Answer from the drawing. Dimensions are ordinates in mm from the lowest x, y and z of the part. A direction names the side the tool comes from. Give positions to 0.01 mm unless a question says otherwise; leave off trailing zeros. Write each loop counter-clockwise with the first axis right and the second up, starting at its lowest first coordinate (ties: lowest second). Pieces come first, ordered by that corner, then holes. Notation, with made-up numbers: M 23.5,50 L 48.5,50 A13 ccw 48.5,68 Z; hole C 9.5,37.5 d7. An arc over 180 degrees is marked long. Answer as a JSON object with one key per item and string values.
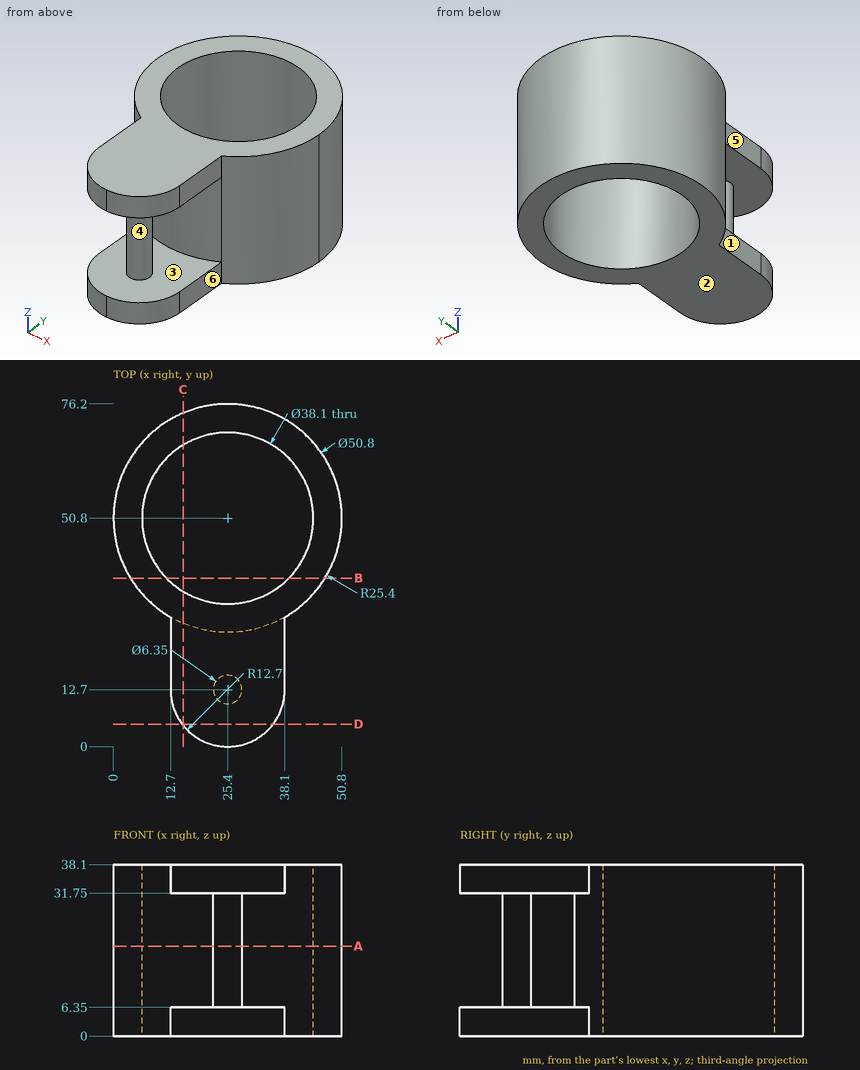
1. A cutting plane is placed at D-D, the plane y = 5. Give the vertices of the cut face in (x, z).
Verdict:
{"outline": "M 15.3,0 L 35.5,0 L 35.5,6.35 L 15.3,6.35 Z; M 15.3,31.75 L 35.5,31.75 L 35.5,38.1 L 15.3,38.1 Z"}
2. A cutting plane is placed at B-B, the plane y = 37.5. Give the vertices of the cut face in (x, z).
Verdict:
{"outline": "M 3.76,0 L 11.76,0 L 11.76,38.1 L 3.76,38.1 Z; M 39.04,0 L 47.04,0 L 47.04,38.1 L 39.04,38.1 Z"}
3. Consider line 1 along Y through (x, z) = (25.4, 11) (3 decimals); line 2 along Y through (x, z) = (25, 29); line 3 along Z through (x, y) = (30, 22.5). Determine where each line is inside the solid, lowest interval first.
Verdict:
{"line 1": "y = 9.525 to 15.875, 25.4 to 31.75, 69.85 to 76.2", "line 2": "y = 9.55 to 15.85, 25.4 to 31.75, 69.85 to 76.2", "line 3": "z = 0 to 6.35, 31.75 to 38.1"}
4. A cutting plane is placed at A-A, the plane z = 20. Give the vertices of the cut face in (x, y) (3 decimals), plus the area to 3 significant figures.
Verdict:
{"outline": "M 12.7,28.803 A25.4 ccw 38.1,28.803 A25.4 ccw long Z; C 25.4,12.7 d6.35; hole C 25.4,50.8 d38.1", "area": "918 mm2"}
5. A cutting plane is placed at C-C, the plane x = 15.5. Give the vertices of the cut face in (y, z).
Verdict:
{"outline": "M 4.75,0 L 34.52,0 L 34.52,38.1 L 4.75,38.1 L 4.75,31.75 L 27.41,31.75 L 27.41,6.35 L 4.75,6.35 Z; M 67.08,0 L 74.19,0 L 74.19,38.1 L 67.08,38.1 Z"}
6. The mould has two halves that part along Z. Classify the marked faces 1, 2 and 3: released by +Z, released by -Z, zero draft, split by the parting line, or undercut.
Verdict:
{"face 1": "zero draft", "face 2": "released by -Z", "face 3": "undercut"}
7. Flat-ended cylindrical pins translate along their axes: pin 1 (5 mm diameter, centred on y = 17.5, z = 33.5, fed in from -X); pin 2 (10 mm diameter, centred on x = 12, z = 30.5, fed in from +Y); pin 3 (8 mm diameter, centred on y = 13, z = 4, fed in from +X). Find the tip coordinate at first contact, or state that the pin passes through.
Verdict:
{"pin 1": "stops at x = 12.7", "pin 2": "stops at y = 74.77", "pin 3": "stops at x = 38.1"}
8. For the marked faces 4, 5 and 6, determine the directions among +Z, -Z, +X, -X, +Y, -Y from which every point of the face is accessible in a straight line to the end or side of a thin tool.
Verdict:
{"face 4": "none", "face 5": "+Z, -Z, -X, -Y", "face 6": "+Z, -Z, +X, -Y"}
